Here's the drawing with two shaded views (mm, measured from the low corner). I have some questions. Give positions to 0.01 mm unless a question says otherwise; leave off trailing zeros. Loops run counter-clockwise (first coordinate to the right, second up) from the corner with the lowest first, then second, coordinate; pieces in that order, holes last. Notation, with made-up numbers: M 34.25,-2.5 L 47.25,-2.5 A6 ccw 47.25,3.5 Z; hole C 61,-7 d9. An arc over 180 degrees is marked long. Use a Markdown table: item, result. Add a question column.
1) Suppose I cut it at B-B on y = 1.4. List the corners of the cut face in (x, z) for me, and give its area (3 significant figures).
2) If I drill on line 1 along X through (y, z) = (1.15, 202.5); line 2 along Z through (x, y) = (161, 0.65); line 3 along Z through (x, y) = (136, 2.25), over which ranges is the centre line in solid material (lowest first)? Write a range as [from, to].
3) Suppose I cut it at C-C on z = 169. List the corners of the cut face in (x, y) for me.
4) Suppose I cut it at A-A on x = 252. List the corners of the cut face in (y, z) for me, and give its area (3 significant figures).
5) Will this pin go through, and if not, where does the flat tip stop? pin 1 Ø1 at (y, z) = (0.5, 136.5) entering from -X.
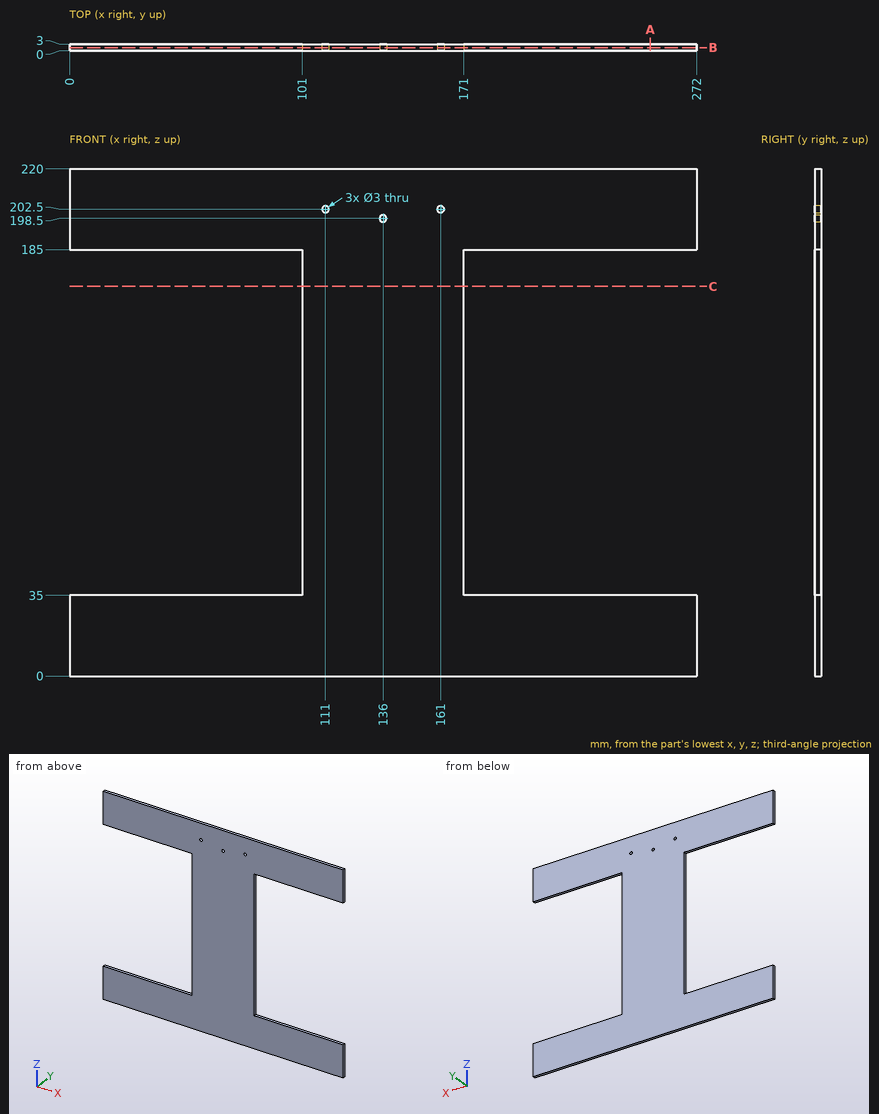
Answer block:
| question | item | result |
|---|---|---|
| 1 | outline | M 0,0 L 272,0 L 272,35 L 171,35 L 171,185 L 272,185 L 272,220 L 0,220 L 0,185 L 101,185 L 101,35 L 0,35 Z; hole C 111,202.5 d3; hole C 136,198.5 d3; hole C 161,202.5 d3 |
| 1 | area | 29,500 mm^2 |
| 2 | line 1 | x = [0, 109.5], [112.5, 159.5], [162.5, 272] |
| 2 | line 2 | z = [0, 201], [204, 220] |
| 2 | line 3 | z = [0, 197], [200, 220] |
| 3 | outline | M 101,0 L 171,0 L 171,3 L 101,3 Z |
| 4 | outline | M 0,0 L 3,0 L 3,35 L 0,35 Z; M 0,185 L 3,185 L 3,220 L 0,220 Z |
| 4 | area | 210 mm^2 |
| 5 | pin 1 | stops at x = 101 |
